Build history of the part. All positions in model axes, mm. A direction names the side the tool comes from. Coordinates: 2 decimals unless noted, no trailing zeros. Write each loop counter-clockwise with the first axis right and the second up, starting at its lowest first coordinate (ties: lowest second). Pieces come first, ordered by that corner, then holes.
from build123d import *

# Parameters (mm, degrees)
F0_W     = 83.355368
F0_H     = 45.16244
F1_DEPTH = 56.388
F3_DEPTH = 25.4
F5_DEPTH = 25.4


with BuildPart() as f1:
    # F0 (on Top) → F1 (new body)
    with BuildSketch(Plane.XY):
        Rectangle(F0_W, F0_H)
    extrude(amount=F1_DEPTH)

    # F2 (on face) → F3 (cut)
    with BuildSketch(Plane.XZ.offset(22.58122)):
        Polygon((41.677684, 56.388), (-19.654024, 56.388), (41.677684, 0), align=None)
    extrude(amount=-F3_DEPTH, mode=Mode.SUBTRACT)

    # F4 (on face) → F5 (cut)
    with BuildSketch(Plane.XZ.offset(-2.81878)):
        Polygon((41.677684, 56.388), (20.490363, 56.388), (41.677684, 37.021209), align=None)
    extrude(amount=-F5_DEPTH, mode=Mode.SUBTRACT)


solid = f1.part
(1) Slice it at A-A, the plane y = 18. List the corners of the cut face in (x, z), and give its area (3 significant figures).
(2) Flat gauge pins, fed straight in: P1, Ø4, axis at x = -1.5, y = -11, coming from the -Z side; P2, Ø5, axis at x = 31.5, z = 47, coming from the -Y side. Where does each tip first touch, or does it go through?
(3) Slice it at D-D, the plane y = -4. List the corners of the cut face in (x, z).
(4) Slice it at B-B, the plane z = 53.5. List the corners of the cut face in (x, y), and give its area (3 significant figures).
(5) Probe L1, parallel to Y at x = 1.5, z = 51; L2, parallel to Z at x = -15.5, y = -17.5; L3, parallel to Z at x = -5, y = -12. List the from-to ranges inside material, lowest first.
(6) Slice it at C-C, the plane x = -5. List the corners of the cut face in (y, z).
(7) 3-axis set-ups, long thin cutter, end or side, ignore diameter. For faces 1 (the flat face through (-1, 0, 0)), 2 (the flat face through (17, 2.819, 35)): which of +Z, -Z, +X, -X, +Y, -Y reach the whole face in a straight line?
Results:
1. outline: (-41.68, 0) - (41.68, 0) - (41.68, 37.02) - (20.49, 56.39) - (-41.68, 56.39) - close
1. area: 4,500 mm2
2. P1: stops at z = 0
2. P2: stops at y = 2.82
3. outline: (-41.68, 0) - (41.68, 0) - (-19.65, 56.39) - (-41.68, 56.39) - close
4. outline: (-41.68, -22.58) - (-16.51, -22.58) - (-16.51, 2.82) - (23.65, 2.82) - (23.65, 22.58) - (-41.68, 22.58) - close
4. area: 1,930 mm2
5. L1: y = 2.82 to 22.58
5. L2: z = 0 to 52.57
5. L3: z = 0 to 42.92
6. outline: (-22.58, 0) - (22.58, 0) - (22.58, 56.39) - (2.82, 56.39) - (2.82, 42.92) - (-22.58, 42.92) - close
7. face 1: -Z, +X, -X, +Y, -Y
7. face 2: +Z, +X, -Y
